Could you check a few things on this model? Use its own coordinates, in mm. A direction names the side the tool comes from. Round coordinates to 2 decimals unless told otherwise and drop trailing zeros. Write each loop counter-clockwise with the first axis right and the second up, starting at its lowest first coordinate (ties: lowest second). Pieces come first, ordered by that corner, then holes. Notation, with made-up numbers: (-12, 28.5) -> (0, 28.5) arc R14 cw to (0, 48.5) -> close; hole circle Ø1 at (58.25, 35). An arc over 180 degrees is marked (long way). Answer in a Markdown table with one row per item. Add a question column.
```python
from build123d import *

# Parameters (mm, degrees)
BOSS_EXTRUDE1_DEPTH = 6.88
SKETCH3_R           = 4
BOSS_EXTRUDE2_DEPTH = 64
SKETCH4_R           = 4
CUT_EXTRUDE1_DEPTH  = 0.7
CUT_EXTRUDE1_TAPER  = -45
CHAMFER1_SIZE       = 0.7


with BuildPart() as part:
    # Sketch1 → Revolve1 (revolve)
    with BuildSketch(Plane.XY):
        with BuildLine():
            Line((0, 0), (8.5, 0))
            ThreePointArc((8.5, 0), (8.580384758, 0.3), (8.5, 0.6))
            Line((8.5, 0.6), (5.680922138, 1.62606043))
            Line((5.680922138, 1.62606043), (0, 1.62606043))
            Line((0, 1.62606043), (0, 0))
        make_face()
    revolve(axis=Axis((0, 1.62606043, 0), (0, -1, 0)))

    # Sketch2 → Boss-Extrude1 (add)
    with BuildSketch(Plane(origin=(0, 1.62606043, 0), x_dir=(1, 0, 0), z_dir=(0, 1, 0))):
        Polygon((6, 0), (3, 5.196152423), (-3, 5.196152423), (-6, 0), (-3, -5.196152423), (3, -5.196152423), align=None)
    extrude(amount=BOSS_EXTRUDE1_DEPTH)

    # Sketch3 → Boss-Extrude2 (add)
    with BuildSketch(Plane.XZ):
        Circle(SKETCH3_R)
    extrude(amount=BOSS_EXTRUDE2_DEPTH)

    # Sketch4 → Cut-Extrude1 (cut)
    with BuildSketch(Plane.XZ.offset(64)):
        Circle(SKETCH4_R)
    extrude(amount=-CUT_EXTRUDE1_DEPTH, taper=CUT_EXTRUDE1_TAPER, mode=Mode.SUBTRACT)

    # Chamfer1
    chamfer1_edges = [part.edges().sort_by_distance(p)[0] for p in [
        (-4, -63.3, 0),
    ]]
    chamfer(chamfer1_edges, length=CHAMFER1_SIZE)


solid = part.part
```
(1) If we mould it in two halves opening along X, with no side actions, what happens to faces 6 (the face through (0, 5, 5.196)), 7 (the face through (-0.867, -30.862, -3.905)), 8 (the face through (4.5, 5, -2.6)), 9 (the face through (-4.5, 5, -2.6))? For each: pulls with the +X half, pulls with the -X half, needs draft (parallel to the pull), parting line crosses it, or undercut.
(2) Suppose I cut it at A-A, the plane x = 0. Please give me the cut outline in (y, z).
(3) For P1, Ø1.8, axis at x = -0.5, y = 4, coming from the -Z side; P2, Ø1.5, axis at x = -2, z = -5, coming from the -Y side; P3, Ø10, axis at x = 1.5, y = -49.5, coming from the +Z side, each with a flat end and sliding along its axis, tell me the tip position at first contact or that it passes through.
(4) Suppose I cut it at B-B, the plane y = -40. Please give me the cut outline in (x, z).
(5) I need wall thicknesses on L1, parallel to Y at x = 5.5, z = -1.5; L2, parallel to Z at x = -2.25, y = -16; L3, parallel to X at y = -33.5, z = -1. Which ranges of each line are inside material? Lowest first, please.
(6) On a 3-axis mill with a long thin cutter (end or side, diameter ignored), from which of +Z, -Z, +X, -X, +Y, -Y can I reach the whole of each face in a straight line? I mean faces 1 (the face through (-4.5, 5, 2.6)), 2 (the face through (4.7, 1.626, -2.7)), 3 (the face through (0, 5, -5.196)), 4 (the face through (-4, 0, -2)), 5 (the face through (4.5, 5, 2.6)). Say none if no direction works.
Response:
| question | item | result |
|---|---|---|
| 1 | face 6 | needs draft |
| 1 | face 7 | parting line crosses it |
| 1 | face 8 | pulls with the +X half |
| 1 | face 9 | pulls with the -X half |
| 2 | outline | (-63.3, -3.3) -> (-62.6, -4) -> (0, -4) -> (0, -8.5) arc R0.6 ccw to (0.6, -8.5) -> (1.63, -5.68) -> (1.63, -5.2) -> (8.51, -5.2) -> (8.51, 5.2) -> (1.63, 5.2) -> (1.63, 5.68) -> (0.6, 8.5) arc R0.6 ccw to (0, 8.5) -> (0, 4) -> (-62.6, 4) -> (-63.3, 3.3) -> close |
| 3 | P1 | z = -5.2 |
| 3 | P2 | y = 0 |
| 3 | P3 | z = 4 |
| 4 | outline | circle Ø8 at (0, 0) |
| 5 | L1 | 0 to 1.62 |
| 5 | L2 | -3.31 to 3.31 |
| 5 | L3 | -3.87 to 3.87 |
| 6 | face 1 | +Z, -X, +Y |
| 6 | face 2 | -Z, +X, +Y |
| 6 | face 3 | -Z, +X, -X, +Y |
| 6 | face 4 | -Y |
| 6 | face 5 | +Z, +X, +Y |
